The listing builds one solid part. Answer for the finished solid, in the listing's coordinates (mm). A direction names the side the tool comes from. Coordinates: 2 decimals unless noted, no trailing zeros. Order: outer loops, then holes, each group sorted by start corner. A loop starts at its lowest first (then second) coordinate and runs counter-clockwise, first axis right, second up. Notation, with made-up numbers: (-16, -14) -> (26, -14) arc R16 cw to (26, 1) -> close; hole circle Ø7 at (6, 29.25). An arc over 180 degrees is marked (long way). Answer in a Markdown table with one row per item.
```python
from build123d import *

# Parameters (mm, degrees)
BOSS_EXTRUDE1_DEPTH = 279.4
SKETCH2_R           = 6.35
CUT_EXTRUDE1_DEPTH  = 45.72
SKETCH3_R           = 6.35
CUT_EXTRUDE2_DEPTH  = 45.72
FILLET1_R           = 2.54


with BuildPart() as part:
    # Sketch1 → Boss-Extrude1 (new body)
    with BuildSketch(Plane(origin=(0, 0, 0), x_dir=(1, 0, 0), z_dir=(0, 1, 0))):
        Polygon((-177.8, -228.6), (-31.75, -228.6), (31.75, -228.6), (177.8, -228.6), (177.8, -41.275), (206.375, -41.275), (206.375, -9.525), (177.8, -9.525), (177.8, 228.6), (0, 228.6), (0, 257.175), (-31.75, 257.175), (-31.75, 228.6), (-177.8, 228.6), (-177.8, -9.525), (-206.375, -9.525), (-206.375, -41.275), (-177.8, -41.275), align=None)
    extrude(amount=BOSS_EXTRUDE1_DEPTH)

    # Sketch2 → Cut-Extrude1 (cut)
    with BuildSketch(Plane.XY.offset(41.275)):
        with Locations((-193.04, 38.1)):
            Circle(SKETCH2_R)
        with Locations((-193.04, 76.2)):
            Circle(SKETCH2_R)
        with Locations((-193.04, 114.3)):
            Circle(SKETCH2_R)
        with Locations((-193.04, 152.4)):
            Circle(SKETCH2_R)
        with Locations((-193.04, 190.5)):
            Circle(SKETCH2_R)
        with Locations((-193.04, 228.6)):
            Circle(SKETCH2_R)
        with Locations((-193.04, 266.7)):
            Circle(SKETCH2_R)
        with Locations((193.04, 266.7)):
            Circle(SKETCH2_R)
        with Locations((193.04, 228.6)):
            Circle(SKETCH2_R)
        with Locations((193.04, 190.5)):
            Circle(SKETCH2_R)
        with Locations((193.04, 152.4)):
            Circle(SKETCH2_R)
        with Locations((193.04, 114.3)):
            Circle(SKETCH2_R)
        with Locations((193.04, 76.2)):
            Circle(SKETCH2_R)
        with Locations((193.04, 38.1)):
            Circle(SKETCH2_R)
    extrude(amount=-CUT_EXTRUDE1_DEPTH, mode=Mode.SUBTRACT)

    # Sketch3 → Cut-Extrude2 (cut)
    with BuildSketch(Plane.ZY.offset(31.75)):
        with Locations((-243.84, 38.1)):
            Circle(SKETCH3_R)
        with Locations((-243.84, 76.2)):
            Circle(SKETCH3_R)
        with Locations((-243.84, 114.3)):
            Circle(SKETCH3_R)
        with Locations((-243.84, 152.4)):
            Circle(SKETCH3_R)
        with Locations((-243.84, 190.5)):
            Circle(SKETCH3_R)
        with Locations((-243.84, 228.6)):
            Circle(SKETCH3_R)
        with Locations((-243.84, 266.7)):
            Circle(SKETCH3_R)
    extrude(amount=-CUT_EXTRUDE2_DEPTH, mode=Mode.SUBTRACT)

    # Fillet1
    fillet1_edges = [part.edges().sort_by_distance(p)[0] for p in [
        (-206.375, 139.7, 41.275),
        (-206.375, 139.7, 9.525),
        (-31.75, 139.7, -257.175),
        (0, 139.7, -257.175),
        (206.375, 139.7, 9.525),
        (206.375, 139.7, 41.275),
    ]]
    fillet(fillet1_edges, radius=FILLET1_R)


solid = part.part
```
(1) A cutting plane is placed at D-D, the plane x = 104.5. Determine the outline of the cut face in (y, z).
Check values:
| item | result |
|---|---|
| outline | (0, -228.6) -> (279.4, -228.6) -> (279.4, 228.6) -> (0, 228.6) -> close |
(2) Which of the six approach directions +Z, -Z, +X, -X, +Y, -Y give full straight-line access (tool end or side, diameter ignored) to faces 1 (the flat face through (177.8, 138, 136)), 2 (the flat face through (90, 138, -228.6)), 3 (the flat face through (-177.8, 138, -111))?
Check values:
| item | result |
|---|---|
| face 1 | +Z, +X, +Y, -Y |
| face 2 | -Z, +X, +Y, -Y |
| face 3 | -Z, -X, +Y, -Y |
(3) Flat-ended cylindrical pins translate along their axes: pin 1 (20.5 mm diameter, centred on x = -193.04, y = 38.1, fed in from -Z) (3 decimals); pin 2 (8 mm diameter, centred on x = 21, y = 161.5, fed in from -Z); pin 3 (16.5 mm diameter, centred on y = 114.3, z = -243.84, fed in from -X). Find the tip coordinate at first contact, or state that the pin passes through.
Check values:
| item | result |
|---|---|
| pin 1 | z = 9.525 |
| pin 2 | z = -228.6 |
| pin 3 | x = -31.75 |
(4) Find the intervals of material crossed by line 1 along Z through (x, y) = (115, 163.5); line 2 along X through (y, z) = (70, 201), in increasing order. Write a range as from..to.
Check values:
| item | result |
|---|---|
| line 1 | -228.6..228.6 |
| line 2 | -177.8..177.8 |
(5) A cutting plane is placed at A-A, the plane z = -243.84. Count the separate pieces of the cut face and the enclosed holes in it, then the cut area to 3 significant figures.
Check values:
| item | result |
|---|---|
| separate pieces | 8 |
| enclosed holes | 0 |
| area | 6,050 mm² |
(6) For a pull along X with two mould halves and no side action, classify faces 4 (the flat face through (-31.75, 138, -242)), 5 (the cylindrical face through (188, 262.84, 25.62)), 6 (the cylindrical face through (-16.097, 264.268, -237.974)) as released by +X, released by -X, zero draft, split by the parting line, or undercut.
Check values:
| item | result |
|---|---|
| face 4 | released by -X |
| face 5 | undercut |
| face 6 | zero draft |
